The model under review builds one solid part; all positions refer to its coordinate system, in mm. Coordinates: 2 decimals unless noted, no trailing zeros. Write each loop counter-clockwise with the first axis right and the second up, starting at its lowest first coordinate (ties: lowest second). Pieces come first, ordered by that corner, then holes. Notation, with made-up numbers: (46.5, 13) - (55.5, 13) arc R25 ccw to (55.5, 29) - close; hole circle Ø10 at (50, -20.5). An arc over 180 degrees is marked (long way). Use one line per item in the form item = value. Start each with the question number.
Autodesk Inventor part; units mm, degrees
ref_plane "YZ Plane" through (0, 0, 0) normal (1, 0, 0) x (0, 1, 0)
ref_plane "XZ Plane" through (0, 0, 0) normal (0, 1, 0) x (-1, 0, 0)
ref_plane "XY Plane" through (0, 0, 0) normal (0, 0, 1) x (1, 0, 0)
sketch "Sketch1" plane through (0, 0, 0) normal (0, 1, 0) x (-1, 0, 0)
  line L0 (0, 0) -> (0, -210) construction
  line L1 (4, 0) -> (4, -210)
  line L2 (-4, -210) -> (-4, 0)
  arc A0 (4, 0) -> (-4, 0) centre (0, 0) ccw
  arc A1 (-4, -210) -> (4, -210) centre (0, -210) ccw
  circle A2 centre (0, 0) radius 2.1
  circle A3 centre (0, -210) radius 2.1
  circle A4 centre (-7, -17) radius 2.1
  circle A5 centre (7, -182) radius 2.1
  circle A6 centre (-7, -17) radius 5
  circle A7 centre (7, -182) radius 5
  point P0 (0, -105)
  point P1 (-4, -13)
  point P2 (-4, -21)
  point P3 (4, -178)
  point P4 (4, -186)
  dimension "d0" = 210
  dimension "d1" = 8
  dimension "d2" = 4.2
  dimension "d3" = 4.2
  dimension "d6" = 4.2
  dimension "d7" = 4.2
  dimension "d8" = 3
  dimension "d9" = 3
  dimension "d10" = 10
  dimension "d11" = 10
  dimension "d12" = 17
  dimension "d13" = 182
extrude "Extrusion1" add sketch "Sketch1" along normal blind 5
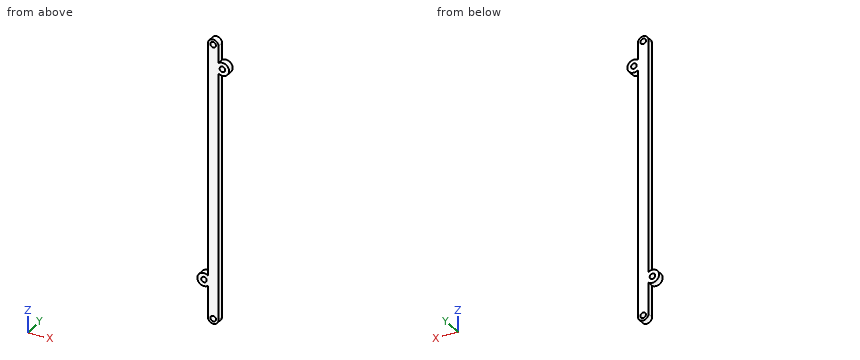
1. For P1, Ø5, axis at x = 0, z = 0, coming from the +Y side; P2, Ø1.5, axis at y = 2, z = -159, coming from the -X side, all flat-tipped, find the tip position at first contact; note any pin that passes through.
2. Take a section at A-A (z = -182). State the section outline as (x, y) points, plus the area to 3 significant figures.
3. Take a section at C-C (x = 7). State the section outline as (y, z) points.
4. For L1, parallel to Z at x = 0, y = 3.6; L2, parallel to Z at x = 7, y = 3.7; L3, parallel to X at y = 1.85, z = -136, list the stretches that pass through material, from the lowest coordinate up.
5. Take a section at B-B (y = 2.25). State the section outline as (x, z) points, plus the area to 3 significant figures.
6. Take a section at D-D (z = -68.5). State the section outline as (x, y) points.
Returned:
q1.P1 = 5
q1.P2 = -4
q2.outline = (-12, 0) - (-9.1, 0) - (-9.1, 5) - (-12, 5) - close; (-4.9, 0) - (4, 0) - (4, 5) - (-4.9, 5) - close
q2.area = 59.0 mm²
q3.outline = (0, -22) - (5, -22) - (5, -19.1) - (0, -19.1) - close; (0, -14.9) - (5, -14.9) - (5, -12) - (0, -12) - close
q4.L1 = -214 to -212.1, -207.9 to -2.1, 2.1 to 4
q4.L2 = -22 to -19.1, -14.9 to -12
q4.L3 = -4 to 4
q5.outline = (-4, -210) arc R4 ccw to (4, -210) - (4, -21) arc R5 ccw (long way) to (4, -13) - (4, 0) arc R4 ccw to (-4, 0) - (-4, -178) arc R5 ccw (long way) to (-4, -186) - close; hole circle Ø4.2 at (-7, -182); hole circle Ø4.2 at (0, -210); hole circle Ø4.2 at (0, 0); hole circle Ø4.2 at (7, -17)
q5.area = 1,810 mm²
q6.outline = (-4, 0) - (4, 0) - (4, 5) - (-4, 5) - close
